from build123d import *

# Parameters (mm, degrees)
SKETCH2_R           = 3.81
BOSS_EXTRUDE1_DEPTH = 1.27
BOSS_EXTRUDE2_DEPTH = 1.27
BOSS_EXTRUDE3_START = 5.842
SKETCH4_R           = 3.81
BOSS_EXTRUDE3_DEPTH = 5.842


with BuildPart() as part:
    # Sketch2 → Boss-Extrude1 (new, symmetric)
    with BuildSketch(Plane(origin=(0, 0, 0), x_dir=(1, 0, 0), z_dir=(0, 1, 0))):
        with Locations(Location((0, 0, 0), (0, 0, 270))):
            Circle(SKETCH2_R)
    extrude(amount=BOSS_EXTRUDE1_DEPTH, both=True)

    # Sketch3 → Boss-Extrude2 (add)
    with BuildSketch(Plane.XZ.offset(1.27)):
        with BuildLine():
            Line((-0.889, 1.0922), (-0.889, -1.0922))
            ThreePointArc((-0.889, -1.0922), (0, -1.397), (0.889, -1.0922))
            Line((0.889, -1.0922), (0.889, 1.0922))
            ThreePointArc((0.889, 1.0922), (0, 1.397), (-0.889, 1.0922))
        make_face()
    extrude(amount=BOSS_EXTRUDE2_DEPTH)

    # Sketch4 → Boss-Extrude3 (add)
    with BuildSketch(Plane(origin=(0, 1.27, 0), x_dir=(1, 0, 0), z_dir=(0, 1, 0)).offset(BOSS_EXTRUDE3_START)):
        with Locations(Location((0, 0, 0), (0, 0, 270))):
            Circle(SKETCH4_R)
        with BuildLine():
            Line((-2.159, 1.9685), (-2.159, -1.9685))
            ThreePointArc((-2.159, -1.9685), (0, -2.54), (2.159, -1.9685))
            Line((2.159, -1.9685), (2.159, 1.9685))
            ThreePointArc((2.159, 1.9685), (0, 2.54), (-2.159, 1.9685))
        make_face(mode=Mode.SUBTRACT)
    extrude(amount=-BOSS_EXTRUDE3_DEPTH)


solid = part.part
For this review, take the finished solid that the model builds, in its own axes (mm). A direction names the side the tool comes from. Give positions to 0.01 mm unless a question says otherwise; leave off trailing zeros. Loops run counter-clockwise (first coordinate to the right, second up) from the corner with the lowest first, then second, coordinate; pieces in that order, holes last. Notation, with made-up numbers: M 61,1.25 L 100,1.25 A15 cw 100,5.25 Z; hole C 51.5,-20 d6. An arc over 180 degrees is marked long. Put each result on its own line as item: value. Start each with the question number.
(1) Add section C-C, the plane y = 6.75. Write out the cut boundary in (x, z), then the cut area to 3 significant figures.
(2) Add section D-D, the plane y = -2. Write out the cut boundary in (x, z), then the cut area to 3 significant figures.
(3) For pin 1 (1 mm diameter, centred on y = -2, z = 0.5, fed in from -X); pin 2 (1 mm diameter, centred on x = 0, z = 1.5, fed in from +Y); pin 3 (1.5 mm diameter, centred on x = -3, z = 1.5, fed in from -Y), all flat-tipped, find the tip position at first contact; note any pin that passes through.
(4) Add section B-B, the plane z = 0. Write out the cut boundary in (x, y), then the cut area to 3 significant figures.
(5) Machinability: for faces 1 (the flat face through (2.159, 4, 0)), 2 (the flat face through (-0.889, -2, 0)), 3 (the cylindrical face through (0.013, -1.896, 1.397)), which of the approach directions +Z, -Z, +X, -X, +Y, -Y give a long, thin tool a straight path to every point of the face, cutting with its end or side? Answer none if there is none.
(6) Add section A-A, the plane x = 0. Write out the cut boundary in (y, z).
(7) The part is to be moulded in two halves that separate along X. For faces 4 (the flat face through (-2.159, 4, 0)), 5 (the cylindrical face through (-0.013, -1.896, -1.397)), 6 (the flat face through (0, 1.27, 0)), 7 (the flat face through (0.889, -2, 0)), say which applies: +X half, -X half, draft (parallel to the pull), parting line (faces both ways), or undercut.
(8) Wall thickness on L1, parallel to Y at x = 1.5, z = 1.25; L2, parallel to Y at x = -0.5, z = -1; L3, parallel to Z at x = 1.75, y = 3.25: over which ranges is each line inside the solid? List them lowest first.
Result:
1. outline: C 0,0 d7.62; hole M -2.16,-1.97 A4.36 ccw 2.16,-1.97 L 2.16,1.97 A4.36 ccw -2.16,1.97 Z
1. area: 25.3 mm^2
2. outline: M -0.89,-1.09 A1.45 ccw 0.89,-1.09 L 0.89,1.09 A1.45 ccw -0.89,1.09 Z
2. area: 4.62 mm^2
3. pin 1: stops at x = -0.89
3. pin 2: stops at y = 1.27
3. pin 3: stops at y = -1.27
4. outline: M -3.81,-1.27 L -0.89,-1.27 L -0.89,-2.54 L 0.89,-2.54 L 0.89,-1.27 L 3.81,-1.27 L 3.81,7.11 L 2.16,7.11 L 2.16,1.27 L -2.16,1.27 L -2.16,7.11 L -3.81,7.11 Z
4. area: 40.9 mm^2
5. face 1: +Y
5. face 2: +Z, -Z, -X, -Y
5. face 3: +Z, -Y
6. outline: M -2.54,-1.4 L -1.27,-1.4 L -1.27,-3.81 L 7.11,-3.81 L 7.11,-2.54 L 1.27,-2.54 L 1.27,2.54 L 7.11,2.54 L 7.11,3.81 L -1.27,3.81 L -1.27,1.4 L -2.54,1.4 Z
7. face 4: undercut
7. face 5: parting line
7. face 6: undercut
7. face 7: +X half
8. L1: y = -1.27 to 1.27
8. L2: y = -2.54 to 1.27
8. L3: z = -3.38 to -2.17, 2.17 to 3.38
